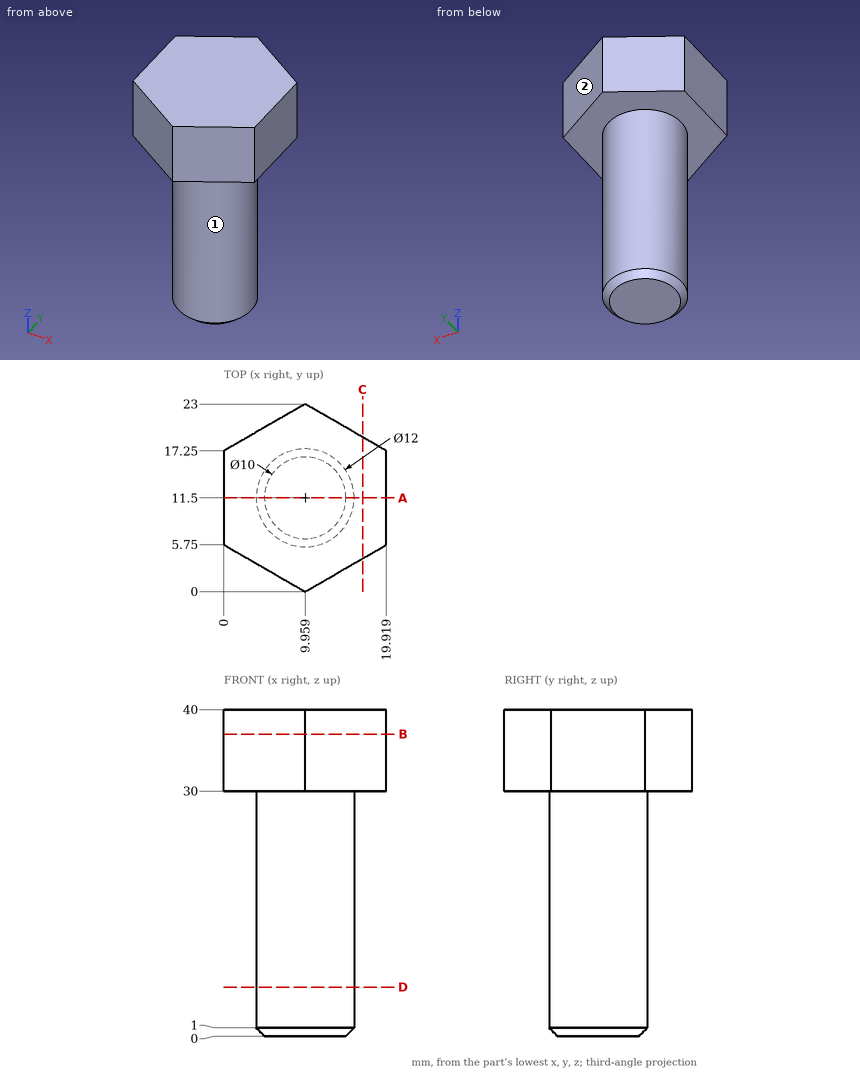
The figure shows three views and two pictorial views of one solid part (mm, origin at its lowest corner). Answer the questions. A direction names the side the tool comes from. Round coordinates to 2 decimals unless told otherwise and drop trailing zeros. Write each loop counter-clockwise with the first axis right and the second up, starting at its lowest first coordinate (ties: lowest second). Pieces come first, ordered by that corner, then holes. Notation, with made-up numbers: (-15, 52) - (19, 52) arc R35 ccw to (19, 86) - close; hole circle Ø11 at (-17.75, -7). An arc over 180 degrees is marked (long way). Use one line per item in the form item = value. Start each with the question number.
Item 1: Find the intervals of material crossed by line 1 (Z direction, x = 1, y = 13.75); line 2 (Y direction, x = 10, z = 19.5); line 3 (Y direction, x = 13, z = 22), in increasing order. Write a range as [from, to].
Item 2: A cutting plane is placed at D-D (z = 6). Write down the section's boundary in (x, y), plus the area to 3 significant figures.
Item 3: A cutting plane is placed at B-B (z = 37). Write down the section's boundary in (x, y).
Item 4: A cutting plane is placed at C-C (x = 17). Write down the section's boundary in (y, z) (1 decimal).
Item 5: Flat-ended cylindrical pins translate along their axes: pin 1 Ø6 at (x, z) = (17, 28.5) entering from -Y (1 decimal); pin 2 Ø6 at (y, z) = (3, 14.5) entering from +X (1 decimal); pin 3 Ø1 at (y, z) = (19, 32.5) entering from +X (1 decimal). Find the tip coordinate at first contact, or state that the pin passes through.
Item 6: A cutting plane is placed at A-A (y = 11.5). Write down the section's boundary in (x, z).
Item 7: A tool of negligible diameter and unlimited length cuts with its end or side. For the marked faces 1 and 2, from which of +Z, -Z, +X, -X, +Y, -Y can it reach the whole face along a straight path? Write none if from no direction.
The answers:
q1.line_1 = [30, 40]
q1.line_2 = [5.5, 17.5]
q1.line_3 = [6.33, 16.67]
q2.outline = circle Ø12 at (9.96, 11.5)
q2.area = 113 mm^2
q3.outline = (0, 5.75) - (9.96, 0) - (19.92, 5.75) - (19.92, 17.25) - (9.96, 23) - (0, 17.25) - close
q4.outline = (4.1, 30) - (18.9, 30) - (18.9, 40) - (4.1, 40) - close
q5.pin_1 = 2.6
q5.pin_2 = 12.4
q5.pin_3 = 17.8
q6.outline = (0, 30) - (3.96, 30) - (3.96, 1) - (4.96, 0) - (14.96, 0) - (15.96, 1) - (15.96, 30) - (19.92, 30) - (19.92, 40) - (0, 40) - close
q7.face_1 = -Z
q7.face_2 = +Z, -Z, +X, +Y
